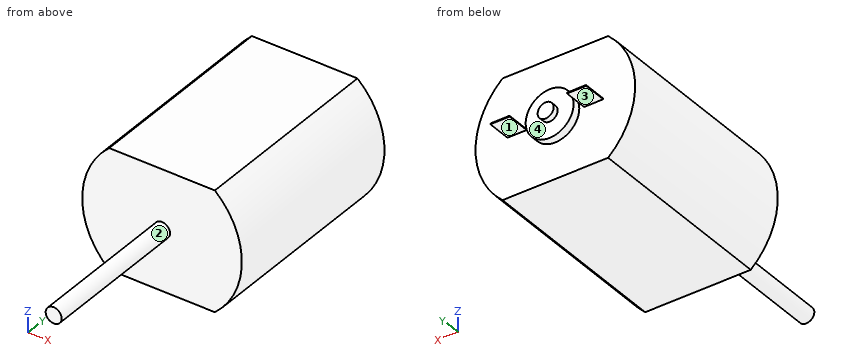
```python
from build123d import *

# Parameters (mm, degrees)
F1_DEPTH = 25
F2_W     = 2.4
F2_H     = 0.1
F3_DEPTH = 3
F4_R     = 3
F4_R_2   = 1
F5_DEPTH = 1
F6_R     = 1
F7_DEPTH = 1.7
F8_R     = 1
F9_DEPTH = 19


with BuildPart() as f1:
    # F0 (on Front) → F1 (new body)
    with BuildSketch(Plane.XZ):
        with BuildLine():
            Line((6.614378, 7.5), (-6.614378, 7.5))
            ThreePointArc((-6.614378, 7.5), (-10, 0), (-6.614378, -7.5))
            Line((-6.614378, -7.5), (6.614378, -7.5))
            ThreePointArc((6.614378, -7.5), (10, 0), (6.614378, 7.5))
        make_face()
    extrude(amount=F1_DEPTH)

    # F2 (on face) → F3 (join)
    with BuildSketch(Plane(origin=(0, 0, 0), x_dir=(-1, 0, 0), z_dir=(0, 1, 0))):
        with Locations((-4.8, 0)):
            Rectangle(F2_W, F2_H)
        with Locations((4.8, 0)):
            Rectangle(F2_W, F2_H)
    extrude(amount=F3_DEPTH)

    # F4 (on face) → F5 (join)
    with BuildSketch(Plane(origin=(0, 0, 0), x_dir=(-1, 0, 0), z_dir=(0, 1, 0))):
        Circle(F4_R)
        Circle(F4_R_2, mode=Mode.SUBTRACT)
    extrude(amount=F5_DEPTH)

    # F6 (on face) → F7 (join)
    with BuildSketch(Plane(origin=(0, 0, 0), x_dir=(-1, 0, 0), z_dir=(0, 1, 0))):
        Circle(F6_R)
    extrude(amount=F7_DEPTH)

    # F8 (on face) → F9 (join)
    with BuildSketch(Plane.XZ.offset(25)):
        Circle(F8_R)
    extrude(amount=F9_DEPTH)


solid = f1.part
```
Verification items for the finished model (mm, model axes). Face numbers are marked on the shaded views. A direction names the side the tool comes from. Give positions to 0.01 mm unless a question says otherwise; leave off trailing zeros. Write each loop counter-clockwise with the first axis right and the second up, starting at its lowest first coordinate (ties: lowest second). Pieces come first, ordered by that corner, then holes. Notation, with made-up numbers: M -11,73.25 L 43,73.25 A11 ccw 43,80.25 Z; hole C 47,18 d1. An arc over 180 degrees is marked long. One line per question, with ' | ' between items.
1) Section check D-D on x = -2.5. Enter the section's corners in (y, z).
Result:
outline: M -25,-7.5 L 0,-7.5 L 0,-1.66 L 1,-1.66 L 1,1.66 L 0,1.66 L 0,7.5 L -25,7.5 Z
2) Section check C-C on y = -23. Enter the section's corners in (x, z).
Result:
outline: M -6.61,-7.5 L 6.61,-7.5 A10 ccw 6.61,7.5 L -6.61,7.5 A10 ccw Z
3) Section check A-A on x = 0. Enter the section's corners in (y, z).
Result:
outline: M -44,-1 L -25,-1 L -25,-7.5 L 0,-7.5 L 0,-3 L 1,-3 L 1,-1 L 1.7,-1 L 1.7,1 L 1,1 L 1,3 L 0,3 L 0,7.5 L -25,7.5 L -25,1 L -44,1 Z
4) Gauge pin test, flat ends, axial feed: pin 1 Ø5 at (x, z) = (2.5, 4.5) entering from -Y; pin 2 Ø2.5 at (x, y) = (4.5, 1.5) entering from -Z; pin 3 Ø1.2 at (x, y) = (-4.5, 1) entering from +Z. Record the tip position at first contact, or that the pin passes through.
Result:
pin 1: stops at y = -25 | pin 2: stops at z = -0.05 | pin 3: stops at z = 0.05
5) Section check B-B on z = 2.25. Enter the section's corners in (x, y), plus the area to 3 significant figures.
Result:
outline: M -9.74,-25 L 9.74,-25 L 9.74,0 L 1.98,0 L 1.98,1 L -1.98,1 L -1.98,0 L -9.74,0 Z | area: 491 mm2
6) Set-up check for the marked faces 1, 2, 3 and 4: record each of +Z, -Z, +X, -X, +Y, -Y from which the full face is reachable in a straight line by a thin tool's end or side.
Result:
face 1: -Z, +X, +Y | face 2: -Y | face 3: -Z, -X, +Y | face 4: +Y
7) Thickness scan on line 1 along Y through (x, z) = (8.5, 2); line 2 along Y through (x, z) = (1.75, 2); line 3 along Z through (x, y) = (7.5, -8). Record the ranges inside material, lowest first. Write a range as [from, to].
Result:
line 1: y = [-25, 0] | line 2: y = [-25, 1] | line 3: z = [-6.61, 6.61]
